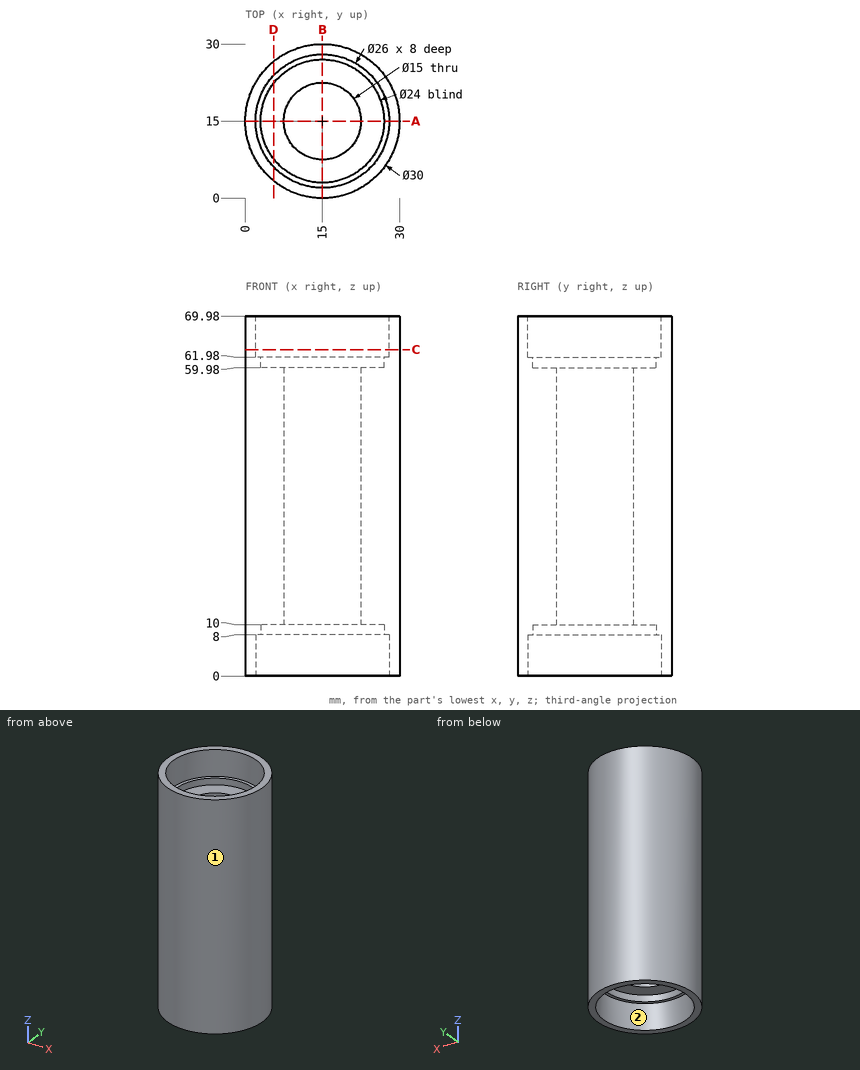
Study the drawing (mm; zero at the part's minimum x, y, z) and answer. Round coordinates to 2 decimals unless told otherwise and drop trailing zeros. Write each loop counter-clockwise with the first axis right and the second up, starting at its lowest first coordinate (ties: lowest second). Pieces come first, ordered by that corner, then holes.
1) A cutting plane is placed at A-A on y = 15. Determine the outline of the cut face in (x, z).
2) Flat-ended cylindrical pins translate along their axes: P1, Ø10, axis at y = 6.5, z = 18.5, coming from the +X side; P2, Ø3, axis at x = 7.5, y = 14, coming from the +Z side; P3, Ø1, axis at x = 23, z = 42.5, coming from the -Y side. Find the tip coordinate at first contact, or state that the pin passes through.
3) A cutting plane is placed at D-D on x = 5.5. Determine the outline of the cut face in (y, z), and give its area (3 significant figures).
4) Determine the mould class of the marked faces 1 and 2 for opening direction Y: pulls with the +Y half, pulls with the -Y half, needs draft (parallel to the pull), parting line crosses it, or undercut.
5) A cutting plane is placed at C-C on z = 63.5. Determine the outline of the cut face in (x, y), and give its area (3 significant figures).
6) Consider probe 1 along Y at (x, z) = (15, 3.75); probe 2 along Y at (x, z) = (15, 61.55); probe 3 along X at (y, z) = (14.5, 61). Determine where each line is inside the solid, lowest interval first.
Entries:
1. outline: (0, 0) - (2, 0) - (2, 8) - (3, 8) - (3, 10) - (7.5, 10) - (7.5, 59.98) - (3, 59.98) - (3, 61.98) - (2, 61.98) - (2, 69.98) - (0, 69.98) - close; (22.5, 10) - (27, 10) - (27, 8) - (28, 8) - (28, 0) - (30, 0) - (30, 69.98) - (28, 69.98) - (28, 61.98) - (27, 61.98) - (27, 59.98) - (22.5, 59.98) - close
2. P1: stops at x = 29.59
2. P2: stops at z = 59.98
2. P3: stops at y = 2.01
3. outline: (3.39, 0) - (6.13, 0) - (6.13, 8) - (7.67, 8) - (7.67, 10) - (22.33, 10) - (22.33, 8) - (23.87, 8) - (23.87, 0) - (26.61, 0) - (26.61, 69.98) - (23.87, 69.98) - (23.87, 61.98) - (22.33, 61.98) - (22.33, 59.98) - (7.67, 59.98) - (7.67, 61.98) - (6.13, 61.98) - (6.13, 69.98) - (3.39, 69.98) - close
3. area: 1,280 mm2
4. face 1: parting line crosses it
4. face 2: undercut
5. outline: circle Ø30 at (15, 15); hole circle Ø26 at (15, 15)
5. area: 176 mm2
6. probe 1: y = 0 to 2, 28 to 30
6. probe 2: y = 0 to 3, 27 to 30
6. probe 3: x = 0.01 to 3.01, 26.99 to 29.99
